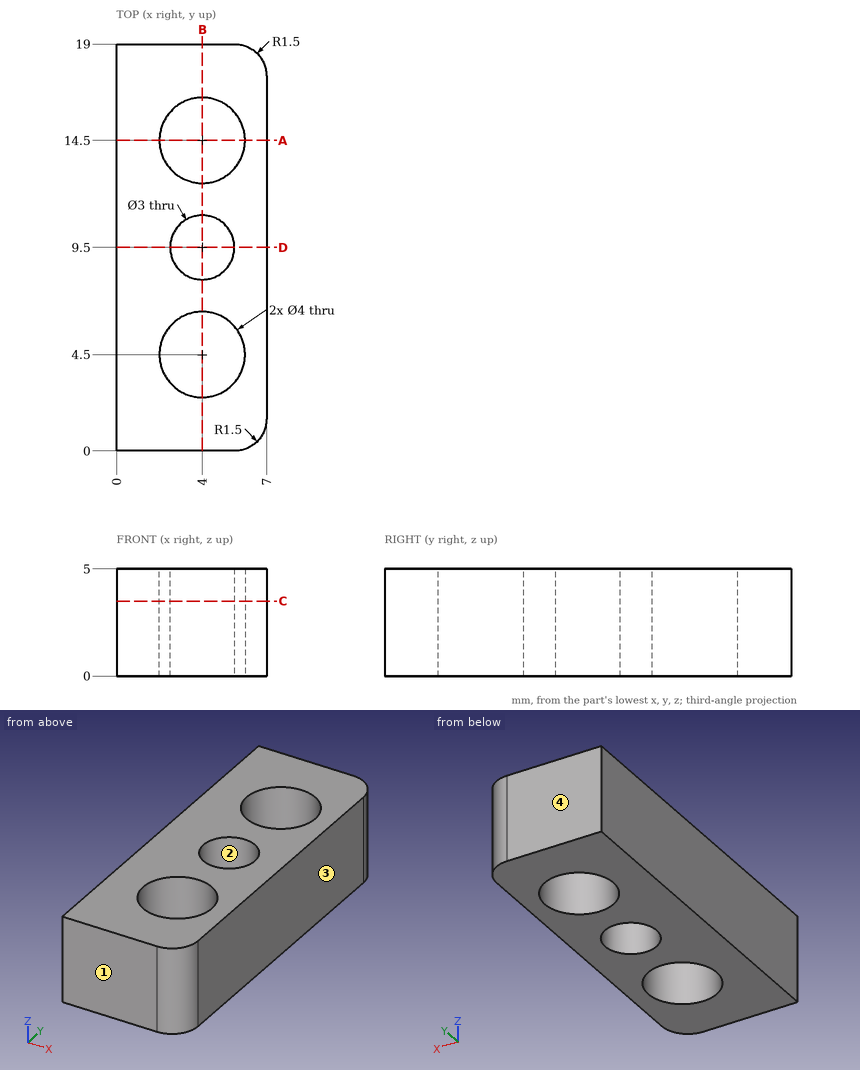
Study the drawing (mm; zero at the part's minimum x, y, z) and answer. Round coordinates to 2 decimals unless told otherwise and drop trailing zeros. Order: outer loops, then holes, each group sorted by start corner. A loop starts at its lowest first (then second) coordinate and runs counter-clockwise, first axis right, second up. Notation, with made-up numbers: (-2, 26) - (53, 26) arc R27 cw to (53, 61) - close; hole circle Ø9 at (31.25, -31.5). An arc over 180 degrees is marked (long way). Use one line per item in the form item = value. Start each with the question number.
(1) The part is cut by section C-C (z = 3.5). Give the vertices of the cut face in (x, y), then the cut area to 3 significant figures.
(2) The part is cut by section B-B (x = 4). Give the vertices of the cut face in (y, z), then the cut area to 3 significant figures.
(3) The part is cut by section A-A (y = 14.5). Give the vertices of the cut face in (x, z), then the cut area to 3 significant figures.
(4) Find the intervals of material crossed by line 1 along Y through (x, z) = (4, 3.75); line 2 along X through (y, z) = (13.75, 3.6); line 3 along X through (y, z) = (6.25, 4.85), in increasing order. Write a range as from..to.
(5) Determine the mould class of the marked faces 1, 2, 3 and 4 for opening direction Y: +Y half, -Y half, draft (parallel to the pull), parting line (faces both ways), or undercut.
(6) The part is cut by section D-D (y = 9.5). Give the vertices of the cut face in (x, z), then the cut area to 3 significant figures.
Checked values:
q1.outline = (0, 0) - (5.5, 0) arc R1.5 ccw to (7, 1.5) - (7, 17.5) arc R1.5 ccw to (5.5, 19) - (0, 19) - close; hole circle Ø4 at (4, 4.5); hole circle Ø4 at (4, 14.5); hole circle Ø3 at (4, 9.5)
q1.area = 99.8 mm^2
q2.outline = (0, 0) - (2.5, 0) - (2.5, 5) - (0, 5) - close; (6.5, 0) - (8, 0) - (8, 5) - (6.5, 5) - close; (11, 0) - (12.5, 0) - (12.5, 5) - (11, 5) - close; (16.5, 0) - (19, 0) - (19, 5) - (16.5, 5) - close
q2.area = 40.0 mm^2
q3.outline = (0, 0) - (2, 0) - (2, 5) - (0, 5) - close; (6, 0) - (7, 0) - (7, 5) - (6, 5) - close
q3.area = 15.0 mm^2
q4.line_1 = 0..2.5, 6.5..8, 11..12.5, 16.5..19
q4.line_2 = 0..2.15, 5.85..7
q4.line_3 = 0..3.03, 4.97..7
q5.face_1 = -Y half
q5.face_2 = undercut
q5.face_3 = draft
q5.face_4 = +Y half
q6.outline = (0, 0) - (2.5, 0) - (2.5, 5) - (0, 5) - close; (5.5, 0) - (7, 0) - (7, 5) - (5.5, 5) - close
q6.area = 20.0 mm^2
